Geometry check sheet. Reference: the model listing, model coordinates, mm. Face numbers are marked on the shaded views. A direction names the side the tool comes from. Coordinates: 2 decimals unless noted, no trailing zeros. Write each loop counter-clockwise with the first axis right and the second up, starting at its lowest first coordinate (ties: lowest second). Pieces come first, ordered by that corner, then holes.
from build123d import *

# Parameters (mm, degrees)
EXTRUDE_1_DEPTH           = 110
CUT_EXTRUDE_2_DEPTH       = 304.47981811
CUT_EXTRUDE_2_DEPTH_BACK  = 304.47981811
SKETCH_2_W                = 90
SKETCH_2_H                = 70
CUT_EXTRUDE_3_DEPTH       = 302.496268634
CUT_EXTRUDE_3_DEPTH_BACK  = 302.496268634
SKETCH_3_R                = 2.5
CUT_EXTRUDE_4_DEPTH       = 302.496268634
CUT_EXTRUDE_4_DEPTH_BACK  = 302.496268634
SKETCH_4_W                = 29.668274831
SKETCH_4_H                = 40
SKETCH_5_R                = 42.5
EXTRUDE_2_DEPTH           = 32.5
SKETCH_6_R                = 38.01
CUT_EXTRUDE_6_DEPTH       = 23.7
SKETCH_7_R                = 32.8
CUT_EXTRUDE_7_DEPTH       = 38.3
SKETCH_9_R                = 1.25
CUT_EXTRUDE_8_DEPTH       = 5
CUT_EXTRUDE_11_DEPTH      = 320.469803837
CUT_EXTRUDE_11_DEPTH_BACK = 320.469803837
SKETCH_10_W               = 30
SKETCH_10_H               = 12
SKETCH_12_R               = 2.5
CUT_EXTRUDE_13_DEPTH      = 10


with BuildPart() as part:
    # 草图1 → 凸台-拉伸1 (new body)
    with BuildSketch(Plane(origin=(0, 0, 0), x_dir=(0, 0, -1), z_dir=(1, 0, 0))):
        with BuildLine():
            Line((0, 20), (260, 20))
            ThreePointArc((260, 20), (280, 0), (260, -20))
            Line((260, -20), (0, -20))
            ThreePointArc((0, -20), (-20, 0), (0, 20))
        make_face()
    extrude(amount=EXTRUDE_1_DEPTH)

    # 草图2 → 切除-拉伸2 (cut, two sides: drawn at the far end of the back side and taken through both)
    with BuildSketch(Plane(origin=(0, 20, 0), x_dir=(1, 0, 0), z_dir=(0, 1, 0)).offset(-CUT_EXTRUDE_2_DEPTH_BACK)):
        with Locations((55, 15)):
            Rectangle(SKETCH_2_W, SKETCH_2_H)
    extrude(amount=CUT_EXTRUDE_2_DEPTH + CUT_EXTRUDE_2_DEPTH_BACK, mode=Mode.SUBTRACT)

    # 草图3 → 切除-拉伸3 (cut, two sides: drawn at the far end of the back side and taken through both)
    with BuildSketch(Plane.ZY.offset(-CUT_EXTRUDE_3_DEPTH_BACK)):
        Circle(SKETCH_3_R)
    extrude(amount=CUT_EXTRUDE_3_DEPTH + CUT_EXTRUDE_3_DEPTH_BACK, mode=Mode.SUBTRACT)

    # 草图4 → 切除-拉伸4 (cut, two sides: drawn at the far end of the back side and taken through both)
    with BuildSketch(Plane(origin=(110, 0, 0), x_dir=(0, 0, -1), z_dir=(1, 0, 0)).offset(-CUT_EXTRUDE_4_DEPTH_BACK)):
        with Locations((267.649236146, 0)):
            Rectangle(SKETCH_4_W, SKETCH_4_H)
    extrude(amount=CUT_EXTRUDE_4_DEPTH + CUT_EXTRUDE_4_DEPTH_BACK, mode=Mode.SUBTRACT)

    # 草图5 → 凸台-拉伸2 (add, symmetric)
    with BuildSketch(Plane(origin=(0, 0, -252.81509873), x_dir=(-1, 0, 0), z_dir=(0, 0, -1))):
        with Locations(Location((-55, 0, 0), (0, 0, 151.927513064))):
            Circle(SKETCH_5_R)
    extrude(amount=EXTRUDE_2_DEPTH, both=True)

    # 草图6 → 切除-拉伸6 (cut)
    with BuildSketch(Plane(origin=(0, 0, -285.31509873), x_dir=(-1, 0, 0), z_dir=(0, 0, -1))):
        with Locations((-55, 0)):
            Circle(SKETCH_6_R)
    extrude(amount=-CUT_EXTRUDE_6_DEPTH, mode=Mode.SUBTRACT)

    # 草图7 → 切除-拉伸7 (cut)
    with BuildSketch(Plane(origin=(0, 0, -261.61509873), x_dir=(-1, 0, 0), z_dir=(0, 0, -1))):
        with Locations((-55, 0)):
            Circle(SKETCH_7_R)
    extrude(amount=-CUT_EXTRUDE_7_DEPTH, mode=Mode.SUBTRACT)

    # 草图9 → 切除-拉伸8 (cut)
    with BuildSketch(Plane(origin=(0, 0, -261.61509873), x_dir=(-1, 0, 0), z_dir=(0, 0, -1))):
        with Locations((-55, 34.5)):
            Circle(SKETCH_9_R)
        with Locations((-41.797421583, 31.873843872)):
            Circle(SKETCH_9_R)
        with Locations((-30.604816049, 24.395183951)):
            Circle(SKETCH_9_R)
        with Locations((-23.126156128, 13.202578417)):
            Circle(SKETCH_9_R)
        with Locations((-20.5, 0)):
            Circle(SKETCH_9_R)
        with Locations((-23.126156128, -13.202578417)):
            Circle(SKETCH_9_R)
        with Locations((-30.604816049, -24.395183951)):
            Circle(SKETCH_9_R)
        with Locations((-41.797421583, -31.873843872)):
            Circle(SKETCH_9_R)
        with Locations((-55, -34.5)):
            Circle(SKETCH_9_R)
        with Locations((-68.202578417, -31.873843872)):
            Circle(SKETCH_9_R)
        with Locations((-79.395183951, -24.395183951)):
            Circle(SKETCH_9_R)
        with Locations((-86.873843872, -13.202578417)):
            Circle(SKETCH_9_R)
        with Locations((-89.5, 0)):
            Circle(SKETCH_9_R)
        with Locations((-86.873843872, 13.202578417)):
            Circle(SKETCH_9_R)
        with Locations((-79.395183951, 24.395183951)):
            Circle(SKETCH_9_R)
        with Locations((-68.202578417, 31.873843872)):
            Circle(SKETCH_9_R)
    extrude(amount=-CUT_EXTRUDE_8_DEPTH, mode=Mode.SUBTRACT)

    # 草图10 → 切除-拉伸11 (cut, two sides: drawn at the far end of the back side and taken through both)
    with BuildSketch(Plane(origin=(0, 50, 0), x_dir=(1, 0, 0), z_dir=(0, 1, 0)).offset(-CUT_EXTRUDE_11_DEPTH_BACK)):
        with Locations((55, 230.078307714)):
            Rectangle(SKETCH_10_W, SKETCH_10_H)
    extrude(amount=CUT_EXTRUDE_11_DEPTH + CUT_EXTRUDE_11_DEPTH_BACK, mode=Mode.SUBTRACT)

    # 草图12 → 切除-拉伸13 (cut)
    with BuildSketch(Plane.ZY):
        with Locations((0, -10)):
            Circle(SKETCH_12_R)
    extrude(amount=-CUT_EXTRUDE_13_DEPTH, mode=Mode.SUBTRACT)


solid = part.part
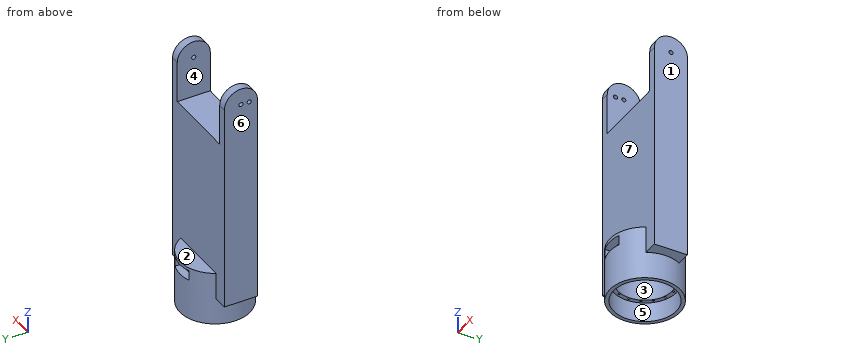
1. Sectioned sample at A-A, the plane z = -92. Record the boundary of the cut face in (x, y).
Computed values:
outline: (0, -20) - (110, -20) - (110, 20) - (0, 20) - close
2. Access from +Z, -Z, +X, -X, +Y, -Y to the whole of each face (thin tool, end or side, straight path). Record for the marked faces 1, 2, 3 and 4.
Computed values:
face 1: +Z, -Z, +X, +Y, -Y
face 2: +Z, +X, -X, +Y
face 3: -Z
face 4: +Z, +Y, -Y
3. Draft check along X on the marked faces 5, 6 and 7. Enter one of: released by +X, released by -X, zero draft, split by the parting line, or undercut.
Computed values:
face 5: undercut
face 6: released by -X
face 7: zero draft
4. Thickness scan on line 1 along X through (y, z) = (-10.5, -28.5); line 2 along Y through (x, z) = (55, -260.2); line 3 along Y through (x, z) = (55, -250). Record the ranges inside material, lowest first.
Computed values:
line 1: x = 0 to 10, 100 to 110
line 2: y = -42.5 to -35.75, -33.25 to -32.8, 32.8 to 33.25, 35.75 to 42.5
line 3: y = -42.5 to -32.8, 32.8 to 42.5
5. Gauge pin test, flat ends, axial feed: pin 1 Ø3 at (x, y) = (30.5, -24) entering from -Z; pin 2 Ø10.5 at (x, y) = (57, 32.5) entering from +Z; pin 3 Ø10 at (x, z) = (16.5, -71.5) entering from +Y. Record the tip position at first contact, or that the pin passes through.
Computed values:
pin 1: stops at z = -261.62
pin 2: stops at z = -220.32
pin 3: stops at y = 20
